from build123d import *

# Parameters (mm, degrees)
F0_R          = 50
F1_DEPTH      = 125
F2_T          = -8
F3_R          = 5
F6_DEPTH      = 10
F6_DEPTH_BACK = 10
F7_R          = 2.5
F8_R          = 2.49999
F9_R          = 4.99999


# Not quite as in the source:
# - a fillet or chamfer that OpenCascade refuses, or shapes differently, is made with other operations: its cross-section is extruded or revolved along the edge and cut away or added
# - a fillet or chamfer is up to 0.001 mm smaller than in the source, because OpenCascade refuses the exact size


with BuildPart() as f1:
    # F0 (on Top) → F1 (new body)
    with BuildSketch(Plane.XY):
        Circle(F0_R)
    extrude(amount=F1_DEPTH)

    # F2
    f2_openings = [f1.faces().sort_by_distance(p)[0] for p in [
        (0, 0, 125),
    ]]
    offset(amount=F2_T, openings=f2_openings)

    # F3
    f3_edges = [f1.edges().sort_by_distance(p)[0] for p in [
        (-50, 0, 125),
    ]]
    fillet(f3_edges, radius=F3_R)

    # F4: fillet of radius 5 on 1 edges, made by hand

    # F4_s1 → F4_t2 (revolve, cut)
    with BuildSketch(Plane.XZ):
        with BuildLine():
            ThreePointArc((45, 125), (42.8166998673, 123.1560370926), (42, 120.417424305))
            Line((42, 120.417424305), (42, 125))
            Line((42, 125), (45, 125))
        make_face()
    revolve(axis=Axis((0, 0, 125), (0, 0, 1)), mode=Mode.SUBTRACT)

    # F5 (on Right) → F6 (join, two sides)
    with BuildSketch(Plane.YZ) as f6_sk:
        with BuildLine():
            ThreePointArc((-49.5038208311, 28.4888988916), (-84.9579082425, 63.4859531194), (-49.5038208311, 98.4830073472))
            Line((-49.5038208311, 98.4830073472), (-49.5038208311, 103.4833755941))
            ThreePointArc((-49.5038208311, 103.4833755941), (-89.9579082425, 63.4859531194), (-49.5038208311, 23.4885306446))
            Line((-49.5038208311, 23.4885306446), (-49.5038208311, 28.4888988916))
        make_face()
    extrude(amount=F6_DEPTH)
    extrude(f6_sk.sketch, amount=-F6_DEPTH_BACK)

    # F7
    f7_edges = [f1.edges().sort_by_distance(p)[0] for p in [
        (10, -89.957908, 63.485953),
    ]]
    fillet(f7_edges, radius=F7_R)

    # F8 (radius 2.5 in the source; OpenCascade refuses exactly that, so slightly less here)
    f8_edges = [f1.edges().sort_by_distance(p)[0] for p in [
        (10, -84.957908, 63.485953),
    ]]
    fillet(f8_edges, radius=F8_R)

    # F9 (radius 5 in the source; OpenCascade refuses exactly that, so slightly less here)
    f9_edges = [f1.edges().sort_by_distance(p)[0] for p in [
        (-10, -89.957908, 63.485953),
    ]]
    fillet(f9_edges, radius=F9_R)


solid = f1.part
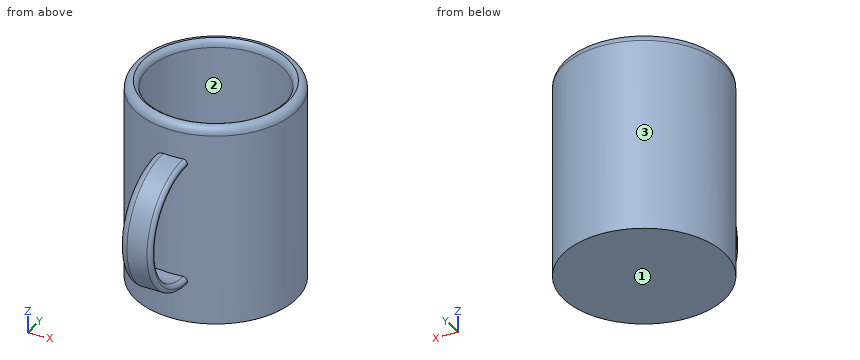
The model under review builds one solid part; all positions refer to its coordinate system, in mm. Face numbers are marked on the shaded views. Round coordinates to 2 decimals unless told otherwise and drop trailing zeros. Loops run counter-clockwise (first coordinate to the right, second up) from the corner with the lowest first, then second, coordinate; pieces in that order, holes last. Notation, with made-up numbers: (-23, 38.5) -> (16, 38.5) arc R23 cw to (16, 54.5) -> close; hole circle Ø10 at (-22, 56.5). An arc over 180 degrees is marked (long way). Answer as CSV lines item,"result".
1) Add section B-B on x = 0. Write out the cut boundary in (y, z), plus the area to 3 significant figures.
Geometry results:
outline,"(-50, 0) -> (50, 0) -> (50, 120) arc R5 ccw to (45, 125) arc R5 ccw to (42, 120.42) -> (42, 8) -> (-42, 8) -> (-42, 120.42) arc R5 ccw to (-45, 125) arc R5 ccw to (-50, 120) -> (-50, 103.49) arc R40 ccw to (-50, 23.49) -> close; hole (-50, 28.49) -> (-50, 98.49) arc R35 ccw to start"
area,"3,240 mm²"
2) To check wall thickness, follow line 1 along Y through (x, z) = (0, 39); line 2 along Z through (x, y) = (4, -24); line 3 along X through (y, z) = (10, 86). State the ranges of each line that lie inside material, in increasing order. Write a range as from..to.
Geometry results:
line 1,"y = -81.59..-74.97, -50..-42, 42..50"
line 2,"z = 0..8"
line 3,"x = -48.99..-40.79, 40.79..48.99"
3) Add section C-C on z = 79. State how many separate pieces and enclosed holes the cut face has, plus the area to 3 significant figures.
Geometry results:
separate pieces,"2"
enclosed holes,"1"
area,"2,410 mm²"
4) For P1, Ø12, axis at x = -13.5, y = -11, coming from the +Z side; P2, Ø1.5, axis at x = -8.5, z = 101.5, coming from the +Y side; P3, Ø8, axis at y = 24.5, z = 39.5, coming from the -X side; P4, Ø19, axis at y = -69, z = 79.5, coming from the +X side, all flat-tipped, find the tip position at first contact; note any pin that passes through.
Geometry results:
P1,"stops at z = 8"
P2,"stops at y = 49.4"
P3,"stops at x = -45.6"
P4,"passes through"
5) Draft analysis for pull direction X (two halves, no side actions). For the marked faces 1, 2 and 3, state which applies: pulls with the +X half, pulls with the -X half, needs draft (parallel to the pull), parting line crosses it, or undercut.
Geometry results:
face 1,"needs draft"
face 2,"undercut"
face 3,"parting line crosses it"
6) Add section A-A on y = 0. Write out the cut boundary in (x, z).
Geometry results:
outline,"(-50, 0) -> (50, 0) -> (50, 120) arc R5 ccw to (45, 125) arc R5 ccw to (42, 120.42) -> (42, 8) -> (-42, 8) -> (-42, 120.42) arc R5 ccw to (-45, 125) arc R5 ccw to (-50, 120) -> close"
